Input: part model. Units: mm. Frame: model coordinates. Coordinates: 2 decimals unless noted, no trailing zeros. Write each loop counter-clockwise with the first axis right and the second up, starting at its lowest first coordinate (ties: lowest second). Pieces come first, ordered by that corner, then holes. Notation, with made-up numbers: (57, 15) - (97, 15) arc R21 ccw to (97, 25) - close; hole circle Ø2 at (-29, -7). An arc over 180 degrees is marked (long way). One line per question, with ' | ' between items. Start each with the question number.
1) Section query C-C on z = 209. Return loops of the section in (x, y).
2) First-contact query: P1, Ø1, axis at x = 3, y = 9, coming from the +Z side; P2, Ø5, axis at x = 4, y = 10, coming from the -Z side. Flat tips, straight axial feed; report the tip coordinate or a pass-through.
3) Line query: line 1 (X direction, y = 3.25, z = 129); line 2 (Y direction, x = 4.25, z = 226). Output: solid intervals per line, ascending.
4) Section query B-B on x = 2.25. Return loops of the section in (y, z), and give its area (3 significant figures).
5) Section query A-A on y = -3.5. Return loops of the section in (x, z).
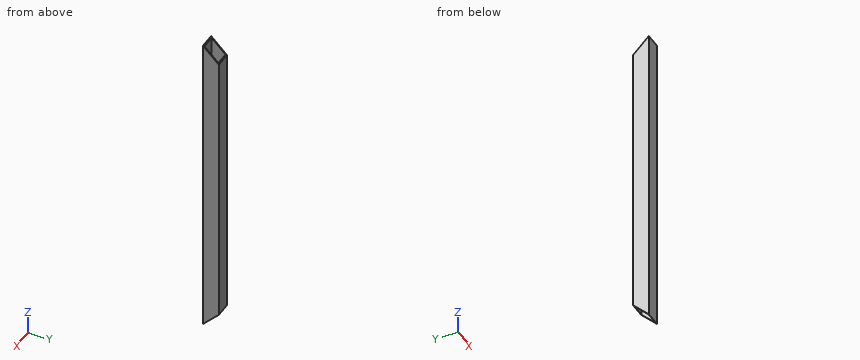
```python
from build123d import *

# Parameters (mm, degrees)
SKETCH1_W           = 25.4
SKETCH1_H           = 25.4
SKETCH1_W_2         = 22.225
SKETCH1_H_2         = 22.225
BOSS_EXTRUDE1_DEPTH = 250
CUT_EXTRUDE1_DEPTH  = 252.607730406


with BuildPart() as part:
    # Sketch1 → Boss-Extrude1 (new, symmetric)
    with BuildSketch(Plane.XY):
        Rectangle(SKETCH1_W, SKETCH1_H)
        Rectangle(SKETCH1_W_2, SKETCH1_H_2, mode=Mode.SUBTRACT)
    extrude(amount=BOSS_EXTRUDE1_DEPTH, both=True)

    # Sketch2 → Cut-Extrude1 (cut, through all)
    with BuildSketch(Plane(origin=(12.7, 0, 0), x_dir=(0, 0, -1), z_dir=(1, 0, 0))):
        Polygon((-250, -12.7), (-250, 12.7), (-224.6, 12.7), align=None)
        Polygon((250, -12.7), (250, 12.7), (224.6, 12.7), align=None)
    extrude(amount=-CUT_EXTRUDE1_DEPTH, mode=Mode.SUBTRACT)


solid = part.part
```
Answer key:
1) outline: (-12.7, -12.7) - (12.7, -12.7) - (12.7, 12.7) - (-12.7, 12.7) - close; hole (-11.11, -11.11) - (11.11, -11.11) - (11.11, 11.11) - (-11.11, 11.11) - close
2) P1: through | P2: z = -226.19
3) line 1: -12.7 to -11.11, 11.11 to 12.7 | line 2: -12.7 to -11.11, 11.11 to 11.3
4) outline: (-12.7, -250) - (-11.11, -248.41) - (-11.11, 248.41) - (-12.7, 250) - close; (11.11, -226.19) - (12.7, -224.6) - (12.7, 224.6) - (11.11, 226.19) - close | area: 1,510 mm²
5) outline: (-12.7, -240.8) - (-11.11, -240.8) - (-11.11, 240.8) - (-12.7, 240.8) - close; (11.11, -240.8) - (12.7, -240.8) - (12.7, 240.8) - (11.11, 240.8) - close
